from build123d import *

# Parameters (mm, degrees)
SKETCH_1_R        = 2.25
SKETCH_1_R_2      = 1.7
SKETCH_1_R_3      = 4.5
SKETCH_1_R_4      = 4
EXTRUDE_1_DEPTH   = 2.5
EXTRUDE_START     = -20
SKETCH_2_W        = 5
SKETCH_2_H        = 61
EXTRUDE_2_DEPTH   = 2
EXTRUDE_2_2_DEPTH = 2
SKETCH_3_W        = 2
SKETCH_3_H        = 29.5
SKETCH_3_H_2      = 24
EXTRUDE_3_DEPTH   = 20
SKETCH_4_W        = 37
SKETCH_4_H        = 2.5
EXTRUDE_4_DEPTH   = 20


with BuildPart() as part:
    # Sketch 1 → Extrude 1 (new body)
    with BuildSketch(Plane(origin=(0, 0, 0), x_dir=(1, 0, 0), z_dir=(0, 1, 0))):
        Polygon((-30, -45.917034388), (30, -45.917034388), (32, -43.917034388), (32, 44.082965612), (30, 46.082965612), (-30, 46.082965612), (-32, 44.082965612), (-32, -43.917034388), align=None)
        with Locations(Location((-15.25, 2.75, 0), (0, 0, 270))):
            Circle(SKETCH_1_R, mode=Mode.SUBTRACT)
        with Locations(Location((-15.25, 33.25, 0), (0, 0, 270))):
            Circle(SKETCH_1_R, mode=Mode.SUBTRACT)
        with Locations(Location((15.25, 2.75, 0), (0, 0, 270))):
            Circle(SKETCH_1_R, mode=Mode.SUBTRACT)
        with Locations(Location((15.25, 33.25, 0), (0, 0, 270))):
            Circle(SKETCH_1_R, mode=Mode.SUBTRACT)
        with Locations(Location((-24, -33, 0), (0, 0, 270))):
            Circle(SKETCH_1_R_2, mode=Mode.SUBTRACT)
        with Locations(Location((-26, -20, 0), (0, 0, 270))):
            Circle(SKETCH_1_R_3, mode=Mode.SUBTRACT)
        with Locations(Location((-26, 20, 0), (0, 0, 270))):
            Circle(SKETCH_1_R_3, mode=Mode.SUBTRACT)
        with Locations(Location((26, -20, 0), (0, 0, 270))):
            Circle(SKETCH_1_R_4, mode=Mode.SUBTRACT)
        with Locations(Location((26, 20, 0), (0, 0, 270))):
            Circle(SKETCH_1_R_4, mode=Mode.SUBTRACT)
        with Locations(Location((24, -33, 0), (0, 0, 90))):
            Circle(SKETCH_1_R_2, mode=Mode.SUBTRACT)
        with Locations(Location((24, 33, 0), (0, 0, 270))):
            Circle(SKETCH_1_R_2, mode=Mode.SUBTRACT)
        with Locations(Location((-24, 33, 0), (0, 0, 90))):
            Circle(SKETCH_1_R_2, mode=Mode.SUBTRACT)
    extrude(amount=EXTRUDE_1_DEPTH)



with BuildPart() as body_2:
    # Sketch 2 → Extrude 2 (new body)
    with BuildSketch(Plane(origin=(0, 0, 0), x_dir=(1, 0, 0), z_dir=(0, 1, 0)).offset(EXTRUDE_START)):
        with Locations((14.5, 0)):
            Rectangle(SKETCH_2_W, SKETCH_2_H)
    extrude(amount=EXTRUDE_2_DEPTH)


with BuildPart() as body_3:
    # Sketch 2 → Extrude 2 2 (new body)
    with BuildSketch(Plane(origin=(0, 0, 0), x_dir=(1, 0, 0), z_dir=(0, 1, 0)).offset(EXTRUDE_START)):
        with Locations((-14.5, 0)):
            Rectangle(SKETCH_2_W, SKETCH_2_H)
    extrude(amount=EXTRUDE_2_2_DEPTH)


with BuildPart() as part_1:
    add(part.part)

    add(body_2.part)  # Extrude 3 merges body 2

    add(body_3.part)  # Extrude 3 merges body 3
    # Sketch 3 → Extrude 3 (add)
    with BuildSketch(Plane(origin=(0, 0, 0), x_dir=(1, 0, 0), z_dir=(0, 1, 0)).offset(EXTRUDE_START)):
        with Locations((17.5, -15.75)):
            Rectangle(SKETCH_3_W, SKETCH_3_H)
        with Locations((-17.5, -15.75)):
            Rectangle(SKETCH_3_W, SKETCH_3_H)
        with Locations((17.5, 18.5)):
            Rectangle(SKETCH_3_W, SKETCH_3_H_2)
        with Locations((-17.5, 18.5)):
            Rectangle(SKETCH_3_W, SKETCH_3_H_2)
    extrude(amount=EXTRUDE_3_DEPTH)

    # Sketch 4 → Extrude 4 (add)
    with BuildSketch(Plane(origin=(0, 0, 0), x_dir=(1, 0, 0), z_dir=(0, 1, 0)).offset(EXTRUDE_START)):
        with Locations((0, -31.25)):
            Rectangle(SKETCH_4_W, SKETCH_4_H)
    extrude(amount=EXTRUDE_4_DEPTH)


solid = part_1.part
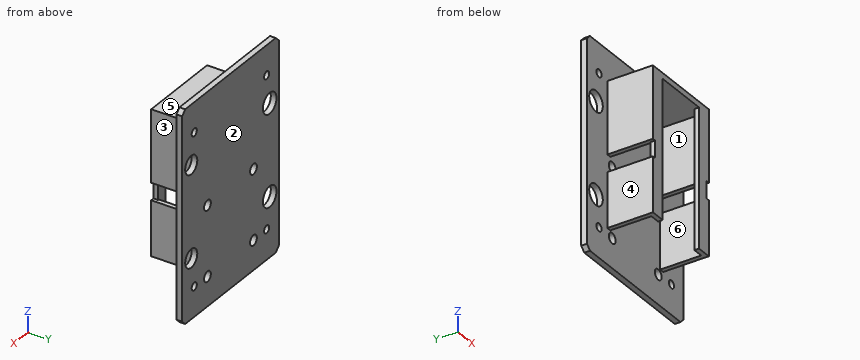
Check sheet for the modelled part. Datum: model origin and axes. Units: mm. Face numbers are marked on the shaded views. A direction names the side the tool comes from. Round coordinates to 2 decimals unless told otherwise and drop trailing zeros. Loops run counter-clockwise (first coordinate to the right, second up) from the corner with the lowest first, then second, coordinate; pieces in that order, holes last.
1. Scan lines: probe 1 along X at (y, z) = (1.25, -33.25); probe 2 along X at (y, z) = (1, -20); probe 3 along X at (y, z) = (1.95, -2.75). Record each from-to range of solid material in increasing order.
2. Gauge pin test, flat ends, axial feed: pin 1 Ø5 at (x, z) = (-15.25, -33.25) entering from +Y; pin 2 Ø3 at (y, z) = (-4, 8.5) entering from -X; pin 3 Ø6 at (x, y) = (4, -6.5) entering from +Z; pin 4 Ø6 at (x, y) = (-10, -4) entering from -Z. Record the tip position at first contact, or that the pin passes through.
3. Sectioned sample at A-A on y = -10. Record the boundary of the cut face in (x, z), and give its area (4 significant figures).
4. Set-up check for the marked faces 4, 5 and 6: record each of +Z, -Z, +X, -X, +Y, -Y from which the full face is reachable in a straight line by a thin tool's end or side.
5. Sectioned sample at C-C on z = 3. Record the boundary of the cut face in (x, y), and give its area (3 significant figures).
6. Mould release check, pull along Y, two halves, no side actions. Record for the marked faces 1, 2 and 3: released by +Y, released by -Y, zero draft, split by the parting line, or undercut.
7. Sectioned sample at B-B on x = -15.25. Record the boundary of the cut face in (y, z), and give its area (4 significant figures).
8. Sectioned sample at D-D on x = -24. Record the boundary of the cut face in (y, z).
Recorded:
1. probe 1: x = -32 to -25.68, -22.32 to -17.5, -13 to 13, 17.5 to 22.32, 25.68 to 32
1. probe 2: x = -32 to -30.5, -21.5 to 22, 30 to 32
1. probe 3: x = -32 to -17.5, -13 to 13, 17.5 to 32
2. pin 1: stops at y = 2.5
2. pin 2: stops at x = -18.5
2. pin 3: stops at z = 32.5
2. pin 4: stops at z = 30
3. outline: (-18.5, -30.5) - (-16.5, -30.5) - (-16.5, -6.5) - (-18.5, -6.5) - close; (-18.5, 1) - (-16.5, 1) - (-16.5, 30) - (16.5, 30) - (16.5, 1) - (18.5, 1) - (18.5, 32.5) - (-18.5, 32.5) - close; (16.5, -30.5) - (18.5, -30.5) - (18.5, -6.5) - (16.5, -6.5) - close
3. area: 304.5 mm2
4. face 4: +Z, -Z, -X, -Y
4. face 5: +Z, +X, -X, -Y
4. face 6: -Z
5. outline: (-32, 0) - (-18.5, 0) - (-18.5, -20) - (-12, -20) - (-12, -18) - (-16.5, -18) - (-16.5, 0) - (16.5, 0) - (16.5, -18) - (12, -18) - (12, -20) - (18.5, -20) - (18.5, 0) - (32, 0) - (32, 2.5) - (-32, 2.5) - close
5. area: 258 mm2
6. face 1: undercut
6. face 2: released by +Y
6. face 3: zero draft
7. outline: (-20, -30.5) - (-18, -30.5) - (-18, 30) - (0, 30) - (0, -0.5) - (2.5, -0.5) - (2.5, 45.92) - (0, 45.92) - (0, 32.5) - (-20, 32.5) - close; (0, -46.08) - (2.5, -46.08) - (2.5, -35.5) - (0, -35.5) - close; (0, -31) - (2.5, -31) - (2.5, -5) - (0, -5) - close
7. area: 378.5 mm2
8. outline: (0, -46.08) - (2.5, -46.08) - (2.5, -34.7) - (0, -34.7) - close; (0, -31.3) - (2.5, -31.3) - (2.5, -24.03) - (0, -24.03) - close; (0, -15.97) - (2.5, -15.97) - (2.5, 15.97) - (0, 15.97) - close; (0, 24.03) - (2.5, 24.03) - (2.5, 31.3) - (0, 31.3) - close; (0, 34.7) - (2.5, 34.7) - (2.5, 45.92) - (0, 45.92) - close
